The listing builds one solid part. Answer for the finished solid, in the listing's coordinates (mm). Coordinates: 2 decimals unless noted, no trailing zeros. Order: outer loops, then holes, each group sorted by start corner. A loop starts at its lowest first (then second) coordinate and runs counter-clockwise, first axis right, second up. Notation, with made-up numbers: (69.25, 26.5) -> (81.25, 26.5) arc R20 cw to (81.25, 53.5) -> close; hole circle Ø2 at (27, 54.5). An arc over 180 degrees is marked (long way). Return JSON: item names as keys, results as strings.
```python
from build123d import *

# Parameters (mm, degrees)
F0_R     = 1.5
F1_DEPTH = 25


with BuildPart() as f1:
    # F0 (on Top) → F1 (new body)
    with BuildSketch(Plane.XY):
        with BuildLine():
            Line((0, -20), (0, 0))
            Line((0, 0), (0, 60))
            Line((0, 60), (-10, 60))
            add(Edge.make_bspline(
                [(-10, 60), (-13.7457798028, 50.0496833938), (-21.165039581, 30.3411079665), (-23.7300116456, 10.047783958), (-25, 0)],
                knots=[0, 0, 0, 0, 0.5048724421, 1, 1, 1, 1], degree=3))
            Line((-25, 0), (-25, -20))
            Line((-25, -20), (0, -20))
        make_face()
        with Locations((-20, -15)):
            Circle(F0_R, mode=Mode.SUBTRACT)
        with Locations((-12, 0)):
            Circle(F0_R, mode=Mode.SUBTRACT)
    extrude(amount=F1_DEPTH)


solid = f1.part
```
Item 1: Find the intervals of material crossed by probe 1 along X at (y, z) = (29.5, 16); probe 2 along X at (y, z) = (6.5, 20.25), in increasing order.
Answer list:
{"probe 1": "-20.12 to 0", "probe 2": "-24.17 to 0"}
Item 2: Determine the mould class of faces 1 (the cylindrical face through (-21.5, -14.93, 12.32)), 2 (the flat face through (-25, -10, 12)), 3 (the flat face through (-13, -20, 12)) for opening direction X: pulls with the +X half, pulls with the -X half, needs draft (parallel to the pull), parting line crosses it, or undercut.
Answer list:
{"face 1": "undercut", "face 2": "pulls with the -X half", "face 3": "needs draft"}
Item 3: The part is cut by section B-B on z = 2. Count the separate pieces of the cut face and the enclosed holes in it, plus the area to 3 significant figures.
Answer list:
{"separate pieces": "1", "enclosed holes": "2", "area": "1,630 mm2"}
Item 4: The part is cut by section A-A on y = -15. Determine the outline of the cut face in (x, z).
Answer list:
{"outline": "(-25, 0) -> (-21.5, 0) -> (-21.5, 25) -> (-25, 25) -> close; (-18.5, 0) -> (0, 0) -> (0, 25) -> (-18.5, 25) -> close"}
Item 5: Flat-ended cylindrical pins translate along their axes: pin 1 (1 mm diameter, centred on y = 39, z = 17, fed in from -X); pin 2 (2 mm diameter, centred on y = 40, z = 12, fed in from -X); pin 3 (10 mm diameter, centred on y = 34, z = 17, fed in from -X). Find the tip coordinate at first contact, or state that the pin passes through.
Answer list:
{"pin 1": "x = -17.61", "pin 2": "x = -17.46", "pin 3": "x = -20.24"}
